The listing builds one solid part. Answer for the finished solid, in the listing's coordinates (mm). Face numbers are marked on the shaded views. Give positions to 0.01 mm unless a question says otherwise; leave off trailing zeros. Loops run counter-clockwise (first coordinate to the right, second up) from the corner with the lowest first, then second, coordinate; pieces in that order, holes last.
Item 1: Section A-A, the plane y = 0 is taken. Give the vertices of the cut face in (x, z), and give its area (3 significant figures).
Item 2: Section D-D, the plane y = -174 is taken. Give the vertices of the cut face in (x, z).
Item 3: Each of these flat-tipped pins is pushed along its axis until it touches: pin 1 Ø2.5 at (x, y) = (-104, 22.5) entering from -Z (3 decimals); pin 2 Ø0.8 at (y, z) = (-123.5, 1) entering from -X; pin 3 Ø0.8 at (x, z) = (-122.5, 0.5) entering from -Y. Where does it stop, or does it pass through?
Item 4: Consider line 1 along X through (y, z) = (-252.5, 0.9); line 2 along Y through (x, z) = (33, 0.45); line 3 along X through (y, z) = (27.5, 0.65). Determine where each line is inside the solid, lowest interval first.
Item 5: The mould has two halves that part along Z. Classify the marked faces 1 and 2: pulls with the +Z half, pulls with the -Z half, needs draft (parallel to the pull), parting line crosses it, or undercut.
Item 6: Section C-C, the plane x = -121.5 is taken. Give the vertices of the cut face in (y, z).
Item 7: Section B-B, the plane z = 0.9 is taken. Give the number of separate pieces and of enclosed holes in the cut face, and give its area (3 significant figures).
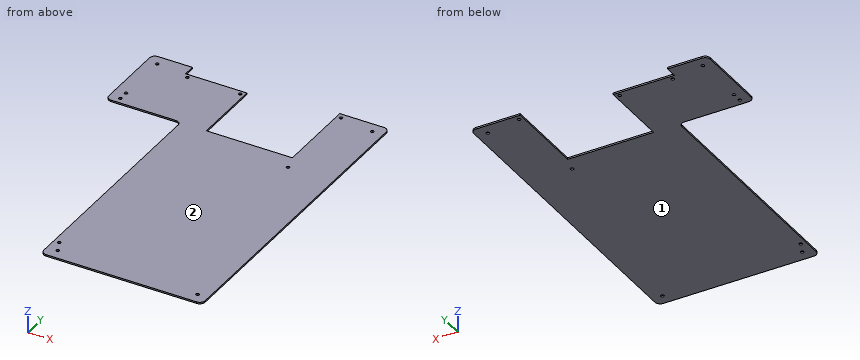
Autodesk Inventor part; units mm, degrees
ref_plane "YZ Plane" through (0, 0, 0) normal (1, 0, 0) x (0, 1, 0)
ref_plane "XZ Plane" through (0, 0, 0) normal (0, 1, 0) x (-1, 0, 0)
ref_plane "XY Plane" through (0, 0, 0) normal (0, 0, 1) x (1, 0, 0)
sketch "スケッチ2" plane through (0, 0, 0) normal (0, 0, 1) x (1, 0, 0)
  line L0 (-70, 37.5) -> (70, 37.5)
  line L1 (75, 32.5) -> (75, -257.5)
  line L2 (70, -262.5) -> (-70, -262.5)
  line L3 (-75, -183.2657) -> (-75, -42.5)
  arc A0 (75, 32.5) -> (70, 37.5) centre (70, 32.5) ccw
  arc A1 (70, -262.5) -> (75, -257.5) centre (70, -257.5) ccw
  line L4 (-75, -257.5) -> (-75, -183.1423)
  arc A2 (-75, -257.5) -> (-70, -262.5) centre (-70, -257.5) ccw
  line L5 (-70, 37.5) -> (-140, 37.5)
  line L6 (-145, 32.5) -> (-145, -32.5)
  line L7 (-140, -37.5) -> (-80, -37.5)
  arc A3 (-140, 37.5) -> (-145, 32.5) centre (-140, 32.5) ccw
  arc A4 (-145, -32.5) -> (-140, -37.5) centre (-140, -32.5) ccw
  arc A5 (-75, -42.5) -> (-80, -37.5) centre (-80, -42.5) ccw
  point P0 (0, 0)
  point P1 (-75, 37.5)
  point P2 (75, -262.5)
  point P3 (75, 37.5)
  point P4 (-75, -262.5)
  point P5 (-75, 0)
  point P6 (0, 37.5)
  point P7 (0, 0)
  point P8 (-145, 0)
  dimension "d1" = 300
  dimension "d24" = 5
  dimension "d49" = 220
  dimension "d50" = 5
  dimension "d51" = 75
extrude "押し出し1" add sketch "スケッチ2" along normal blind 1.5
sketch "スケッチ5" plane through (0, 0, 1.5) normal (0, 0, 1) x (1, 0, 0)
  line L0 (70, 37.5) -> (-140, 37.5)
  line L1 (75, -257.5) -> (75, 32.5)
  line L2 (-70, -262.5) -> (70, -262.5)
  line L3 (-145, 32.5) -> (-145, -32.5)
  line L4 (-140, -37.5) -> (-80, -37.5)
  line L5 (-75, -42.5) -> (-75, -257.5)
  point P0 (-135, 27.5)
  point P1 (65, 27.5)
  point P2 (65, -252.5)
  point P3 (-70, 37.5)
  point P4 (-135, -31.5)
  point P5 (-70, -241.5)
  point P6 (33, -52.5)
  point P7 (33, 32.5)
  point P8 (-55, 22.5)
  point P9 (-135, -22.5)
  point P10 (-65, -252.5)
  point P11 (-104, 22.5)
  dimension "d25" = 10
  dimension "d27" = 10
  dimension "d44" = 80
  dimension "d46" = 85
  dimension "d52" = 10
  dimension "d55" = 10
  dimension "d56" = 10
  dimension "d58" = 21
  dimension "d59" = 5
  dimension "d60" = 15
  dimension "d61" = 69
  dimension "d62" = 5
  dimension "d66" = 54
  dimension "d67" = 49
hole "穴3" at (-135, 27.5, 1.5) at (65, 27.5, 1.5) at (65, -252.5, 1.5) at (-135, -31.5, 1.5) at (-70, -241.5, 1.5) at (-55, 22.5, 1.5) at (33, 32.5, 1.5) at (33, -52.5, 1.5) at (-135, -22.5, 1.5) at (-65, -252.5, 1.5) at (-104, 22.5, 1.5) direction (0, 0, -1) diameter 3 depth 8.1 tip angle 118
sketch "スケッチ6" plane through (0, 0, 1.5) normal (0, 0, 1) x (1, 0, 0)
  point P0 (0, 0)
sketch "スケッチ7" plane through (0, 0, 1.5) normal (0, 0, 1) x (1, 0, 0)
  line L0 (-51, 26.5) -> (-108, 26.5)
  line L1 (-108, 26.5) -> (-108, 37.5)
  line L2 (-108, 37.5) -> (29, 37.5)
  line L3 (29, 37.5) -> (29, -38.5)
  line L4 (-51, 0) -> (-51, 26.5)
  circle A0 centre (-55, 22.5) radius 1.5
  circle A1 centre (-104, 22.5) radius 1.5
  line L5 (70, 37.5) -> (-140, 37.5)
  line L6 (29, -38.5) -> (-51, -38.5)
  line L7 (-51, -38.5) -> (-51, 0)
  point P0 (-25.5, 0)
  dimension "d68" = 4
  dimension "d69" = 4
  dimension "d70" = 4
  dimension "d74" = 76
  dimension "d75" = 80
extrude "押し出し2" cut sketch "スケッチ7" against normal blind 10 contours L0 L1 L2 L3 L6 L7 L4
properties part number "天板"
Worked answers:
1. outline: (-145, 0) - (-51, 0) - (-51, 1.5) - (-145, 1.5) - close; (29, 0) - (75, 0) - (75, 1.5) - (29, 1.5) - close
1. area: 210 mm2
2. outline: (-75, 0) - (75, 0) - (75, 1.5) - (-75, 1.5) - close
3. pin 1: passes through
3. pin 2: stops at x = -75
3. pin 3: stops at y = -37.5
4. line 1: x = -75 to -66.5, -63.5 to 63.5, 66.5 to 75
4. line 2: y = -262.5 to -54, -51 to 31, 34 to 37.5
4. line 3: x = -145 to -136.5, -133.5 to -108, 29 to 63.5, 66.5 to 75
5. face 1: pulls with the -Z half
5. face 2: pulls with the +Z half
6. outline: (-37.5, 0) - (37.5, 0) - (37.5, 1.5) - (-37.5, 1.5) - close
7. separate pieces: 1
7. enclosed holes: 11
7. area: 43,400 mm2
